from build123d import *

# Parameters (mm, degrees)
F1_DEPTH     = 300
F2_W         = 350
F2_H         = 400
F3_DEPTH     = 170
F4_R         = 40
F5_T1_DEPTH  = 170
F5_T4_ANGLE  = 90
F5_T6_ANGLE  = 90
F5_T8_ANGLE  = 90
F5_T10_ANGLE = 90
F7_DEPTH     = 140
F8_R         = 20
F10_DEPTH    = 9
F11_T        = -2.5
F12_DEPTH    = 267.6571849734
F13_R        = 40
F14_DEPTH    = 2.501
F15_R        = 25
F16_DEPTH    = 32.501
F17_R        = 25
F18_DEPTH    = 172.501


# Not quite as in the source:
# - a fillet or chamfer that OpenCascade refuses, or shapes differently, is made with other operations: its cross-section is extruded or revolved along the edge and cut away or added


with BuildPart() as f1:
    # F0 (on Front) → F1 (new body)
    with BuildSketch(Plane.XZ):
        with BuildLine():
            Line((-386, -246), (386, -246))
            ThreePointArc((386, -246), (456.7106781187, -216.7106781187), (486, -146))
            Line((486, -146), (486, 146))
            ThreePointArc((486, 146), (456.7106781187, 216.7106781187), (386, 246))
            Line((386, 246), (-386, 246))
            ThreePointArc((-386, 246), (-456.7106781187, 216.7106781187), (-486, 146))
            Line((-486, 146), (-486, -146))
            ThreePointArc((-486, -146), (-456.7106781187, -216.7106781187), (-386, -246))
        make_face()
    extrude(amount=-F1_DEPTH)

    # F2 (on face) → F3 (cut)
    with BuildSketch(Plane.XZ):
        with Locations((-236, 0)):
            Rectangle(F2_W, F2_H)
    extrude(amount=-F3_DEPTH, mode=Mode.SUBTRACT)

    # F4
    f4_edges = [f1.edges().sort_by_distance(p)[0] for p in [
        (-61, 170, 0),
        (-236, 170, 200),
        (-411, 170, 0),
        (-236, 170, -200),
    ]]
    fillet(f4_edges, radius=F4_R)

    # F5: fillet of radius 100 on 4 edges, made by hand

    # F5_s2 → F5_t1 (join)
    with BuildSketch(Plane.XZ.offset(-170)):
        with BuildLine():
            ThreePointArc((-311, 200), (-381.7106781187, 170.7106781187), (-411, 100))
            Line((-411, 100), (-411, 200))
            Line((-411, 200), (-311, 200))
        make_face()
        with BuildLine():
            ThreePointArc((-311, -200), (-381.7106781187, -170.7106781187), (-411, -100))
            Line((-411, -100), (-411, -200))
            Line((-411, -200), (-311, -200))
        make_face()
        with BuildLine():
            ThreePointArc((-61, 100), (-90.2893218813, 170.7106781187), (-161, 200))
            Line((-161, 200), (-61, 200))
            Line((-61, 200), (-61, 100))
        make_face()
        with BuildLine():
            ThreePointArc((-61, -100), (-90.2893218813, -170.7106781187), (-161, -200))
            Line((-161, -200), (-61, -200))
            Line((-61, -200), (-61, -100))
        make_face()
    extrude(amount=F5_T1_DEPTH)

    # F5_s3 → F5_t4 (revolve)
    with BuildSketch(Plane.XY.offset(-100)):
        with BuildLine():
            ThreePointArc((-101, 170), (-72.7157287525, 158.2842712475), (-61, 130))
            Line((-61, 130), (-61, 170))
            Line((-61, 170), (-101, 170))
        make_face()
    revolve(axis=Axis((-161, 170, -100), (0, 1, 0)), revolution_arc=F5_T4_ANGLE)

    # F5_s5 → F5_t6 (revolve)
    with BuildSketch(Plane.YZ.offset(-161)):
        with BuildLine():
            ThreePointArc((170, 160), (158.2842712475, 188.2842712475), (130, 200))
            Line((130, 200), (170, 200))
            Line((170, 200), (170, 160))
        make_face()
    revolve(axis=Axis((-161, 170, 100), (0, 1, 0)), revolution_arc=F5_T6_ANGLE)

    # F5_s7 → F5_t8 (revolve)
    with BuildSketch(Plane.YZ.offset(-311)):
        with BuildLine():
            ThreePointArc((170, -160), (158.2842712475, -188.2842712475), (130, -200))
            Line((130, -200), (170, -200))
            Line((170, -200), (170, -160))
        make_face()
    revolve(axis=Axis((-311, 170, -100), (0, 1, 0)), revolution_arc=F5_T8_ANGLE)

    # F5_s9 → F5_t10 (revolve)
    with BuildSketch(Plane.XY.offset(100)):
        with BuildLine():
            ThreePointArc((-371, 170), (-399.2842712475, 158.2842712475), (-411, 130))
            Line((-411, 130), (-411, 170))
            Line((-411, 170), (-371, 170))
        make_face()
    revolve(axis=Axis((-311, 170, 100), (0, 1, 0)), revolution_arc=F5_T10_ANGLE)

    # F6 (on face) → F7 (cut)
    with BuildSketch(Plane.XZ):
        with BuildLine():
            ThreePointArc((-11, -100), (49, -160), (109, -100))
            Line((109, -100), (109, 100))
            ThreePointArc((109, 100), (49, 160), (-11, 100))
            Line((-11, 100), (-11, -100))
        make_face()
    extrude(amount=-F7_DEPTH, mode=Mode.SUBTRACT)

    # F8
    f8_edges = [f1.edges().sort_by_distance(p)[0] for p in [
        (49, 140, -160),
        (109, 140, 0),
        (49, 140, 160),
        (-11, 140, 0),
    ]]
    fillet(f8_edges, radius=F8_R)

    # F9 (on face) → F10 (join)
    with BuildSketch(Plane.XZ):
        with BuildLine():
            Line((386, 246), (-386, 246))
            ThreePointArc((-386, 246), (-456.7106781187, 216.7106781187), (-486, 146))
            Line((-486, 146), (-486, -146))
            ThreePointArc((-486, -146), (-456.7106781187, -216.7106781187), (-386, -246))
            Line((-386, -246), (386, -246))
            ThreePointArc((386, -246), (456.7106781187, -216.7106781187), (486, -146))
            Line((486, -146), (486, 146))
            ThreePointArc((486, 146), (456.7106781187, 216.7106781187), (386, 246))
        make_face()
        with BuildLine():
            ThreePointArc((386, 234), (448.2253967444, 208.2253967444), (474, 146))
            Line((474, 146), (474, -146))
            ThreePointArc((474, -146), (448.2253967444, -208.2253967444), (386, -234))
            Line((386, -234), (-386, -234))
            ThreePointArc((-386, -234), (-448.2253967444, -208.2253967444), (-474, -146))
            Line((-474, -146), (-474, 146))
            ThreePointArc((-474, 146), (-448.2253967444, 208.2253967444), (-386, 234))
            Line((-386, 234), (386, 234))
        make_face(mode=Mode.SUBTRACT)
    extrude(amount=F10_DEPTH)

    # F11
    f11_openings = [f1.faces().sort_by_distance(p)[0] for p in [
        (0, 300, 0),
    ]]
    offset(amount=F11_T, openings=f11_openings, kind=Kind.INTERSECTION)

    # F12 (cut): a face of the model
    f12_faces = [f1.faces().sort_by_distance(p)[0] for p in [
        (0, 300, -244.9105744633),
    ]]
    extrude(f12_faces, amount=-F12_DEPTH, mode=Mode.SUBTRACT)

    # F13 (on face) → F14 (cut, through all)
    with BuildSketch(Plane.XZ.offset(-170)):
        with Locations((-236, 100)):
            Circle(F13_R)
    extrude(amount=-F14_DEPTH, mode=Mode.SUBTRACT)

    # F15 (on face) → F16 (cut, through all)
    with BuildSketch(Plane.XZ.offset(-140)):
        with Locations((49, 100)):
            Circle(F15_R)
    extrude(amount=-F16_DEPTH, mode=Mode.SUBTRACT)

    # F17 (on face) → F18 (cut, through all)
    with BuildSketch(Plane.XZ):
        with Locations((-36.2374484539, 197.7449208498)):
            Circle(F17_R)
    extrude(amount=-F18_DEPTH, mode=Mode.SUBTRACT)


solid = f1.part
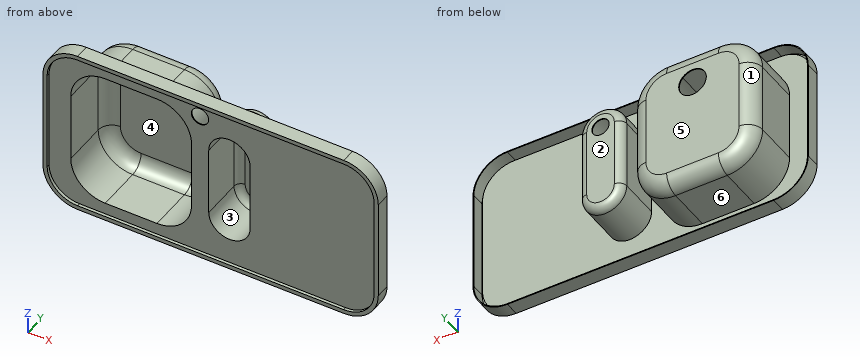
Source: CAD feature listing. Evaluate the final solid. Frame: model axes, mm. Face numbers are marked on the shaded views. A direction names the side the tool comes from. Give positions to 0.01 mm unless a question says otherwise; leave off trailing zeros. Order: outer loops, then holes, each group sorted by start corner. A loop starts at its lowest first (then second) coordinate and runs counter-clockwise, first axis right, second up. Notation, with made-up numbers: (80, 7.5) -> (96, 7.5) arc R31 ccw to (96, 35.5) -> close; hole circle Ø10 at (66, 17). An arc over 180 degrees is marked (long way). Use a Markdown table: item, result.
1) Section query A-A, the plane y = 69.5. Return the cut outline in (x, z).
Answer list:
| item | result |
|---|---|
| outline | (-413.5, -100) arc R102.5 ccw to (-311, -202.5) -> (-161, -202.5) arc R102.5 ccw to (-58.5, -100) -> (-58.5, 100) arc R102.5 ccw to (-161, 202.5) -> (-311, 202.5) arc R102.5 ccw to (-413.5, 100) -> close; (-13.5, -100) arc R62.5 ccw to (111.5, -100) -> (111.5, 100) arc R62.5 ccw to (-13.5, 100) -> close; hole (-411, -100) arc R100 ccw to (-311, -200) -> (-161, -200) arc R100 ccw to (-61, -100) -> (-61, 100) arc R100 ccw to (-161, 200) -> (-311, 200) arc R100 ccw to (-411, 100) -> close; hole (-11, -100) arc R60 ccw to (109, -100) -> (109, 100) arc R60 ccw to (-11, 100) -> close |
2) Contact query for flat-ended pins moving along their axis: P1, Ø1, axis at y = 86.5, z = 1, coming from the +X side; P2, Ø5, axis at x = 357.5, z = -85.5, coming from the +Y side; P3, Ø24, axis at x = 39.5, z = -68, coming from the -Y side. Output: stop coordinate, or through.
Answer list:
| item | result |
|---|---|
| P1 | x = 111.5 |
| P2 | y = 2.5 |
| P3 | y = 140 |
3) Mould query, pull axis X, two halves, no side actions, for the marked faces 1, 2 and 3. Classes: +X half, -X half, draft (parallel to the pull), parting line (faces both ways), or undercut.
Answer list:
| item | result |
|---|---|
| face 1 | -X half |
| face 2 | draft |
| face 3 | undercut |
4) Section query C-C, the plane y = 17. Count the separate pieces of the cut face and the enclosed holes in it, then the cut area to 3 significant figures.
Answer list:
| item | result |
|---|---|
| separate pieces | 3 |
| enclosed holes | 3 |
| area | 12,200 mm² |
5) Ray query, line 1 along X through (y, z) = (57, -86.5); line 2 along Z through (x, y) = (-149, -2); line 3 along Z through (x, y) = (-201, 11). Return the intervals inside material, ascending. Write a range as [from, to].
Answer list:
| item | result |
|---|---|
| line 1 | [-413.5, -411], [-61, -58.5], [-13.5, -11], [109, 111.5] |
| line 2 | [-246, -243.5], [-236.5, -234], [234, 236.5], [243.5, 246] |
| line 3 | [-246, -243.5], [-202.5, -200], [200, 202.5], [243.5, 246] |
6) Reachability of the marked faces 4, 5 and 6 from +Z, -Z, +X, -X, +Y, -Y: full face, straight path, thin tool, end or side. Return the list, or none.
Answer list:
| item | result |
|---|---|
| face 4 | -Y |
| face 5 | +Z, -Z, +X, -X, +Y |
| face 6 | +Y |
